Here's how the part is built. I have some questions about the finished solid (model axes, mm). Face numbers are marked on the shaded views. A direction names the side the tool comes from. Coordinates: 2 decimals unless noted, no trailing zeros. Write each loop counter-clockwise with the first axis right and the second up, starting at its lowest first coordinate (ties: lowest second). Pieces come first, ordered by that corner, then holes.
Item 1: If I drill on line 1 (Z direction, x = 31, y = -0.5); line 2 (X direction, y = -1.5, z = -4.5); line 3 (Z direction, x = 61, y = -1.5), over which ranges is the centre line in solid material (lowest first)?
Item 2: If we section it at C-C (z = -12.5): Please give me the cut outline in (x, y).
Item 3: I'm going to push flat-ended pins straight in: pin 1 Ø1.5 at (x, y) = (28.5, -2) entering from -Z; pin 2 Ø1 at (y, z) = (-2, -12.5) entering from +X; pin 3 Ø3 at (x, y) = (53, -2) entering from +Z. Where does each tip first touch, or does it pass through?
Item 4: For the marked faces 1, 2, 3, 4 and 5, which set-ups out of +Z, -Z, +X, -X, +Y, -Y let a thin tool reach every point of the face, with its end or its side?
Item 5: If we section it at B-B (x = 4.5): Please give me the cut outline in (y, z).
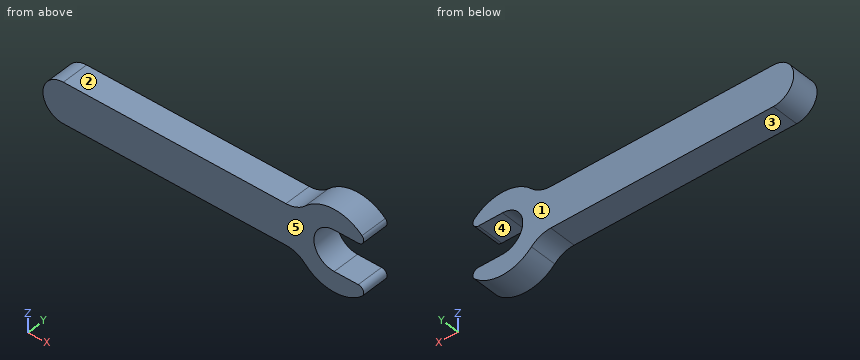
from build123d import *

# Parameters (mm, degrees)
F1_DEPTH = 6.35


with BuildPart() as f1:
    # F0 (on Front) → F1 (new body)
    with BuildSketch(Plane.XZ):
        with BuildLine():
            Line((52.175445, 0), (0, 0))
            ThreePointArc((0, 0), (-4.7752, -4.7752), (0, -9.5504))
            Line((0, -9.5504), (52.175445, -9.5504))
            ThreePointArc((52.175445, -9.5504), (54.631508, -10.044612), (56.705267, -11.45032))
            ThreePointArc((56.705267, -11.45032), (63.295562, -14.298006), (70.001999, -11.735777))
            ThreePointArc((70.001999, -11.735777), (70.316497, -10.341737), (69.135066, -9.5377))
            Line((69.135066, -9.5377), (63.5, -9.5377))
            ThreePointArc((63.5, -9.5377), (58.7375, -4.7752), (63.5, -0.0127))
            Line((63.5, -0.0127), (69.135066, -0.0127))
            ThreePointArc((69.135066, -0.0127), (70.316497, 0.791337), (70.001999, 2.185377))
            ThreePointArc((70.001999, 2.185377), (63.295562, 4.747606), (56.705267, 1.89992))
            ThreePointArc((56.705267, 1.89992), (54.631508, 0.494212), (52.175445, 0))
        make_face()
    extrude(amount=F1_DEPTH)


solid = f1.part
Answer list:
1. line 1: z = -9.55 to 0
1. line 2: x = -4.77 to 58.75
1. line 3: z = -13.97 to -8.83, -0.72 to 4.42
2. outline: (57.93, -6.35) - (69.07, -6.35) - (69.07, 0) - (57.93, 0) - close
3. pin 1: stops at z = -9.55
3. pin 2: stops at x = 69.71
3. pin 3: stops at z = 0.44
4. face 1: +Z, -Z, +X, -X, +Y
4. face 2: +Z, -X, +Y, -Y
4. face 3: -Z, -X, +Y, -Y
4. face 4: +X, +Y, -Y
4. face 5: +Z, -Z, +X, -X, -Y
5. outline: (-6.35, -9.55) - (0, -9.55) - (0, 0) - (-6.35, 0) - close
